Input: part model. Units: mm. Frame: model coordinates. A direction names the side the tool comes from. Round coordinates to 2 decimals unless told otherwise and drop trailing zeros. Order: outer loops, then holes, each group sorted by start corner. A loop starts at its lowest first (then second) coordinate and runs counter-clockwise, first axis right, second up. Notation, with made-up numbers: M 71,-6 L 76,-6 A14 cw 76,1 Z; hole C 73,89 d4. An arc over 180 degrees is marked long. One line per question, with ' | ' between items.
Solid Edge part; units mm, degrees
sketch "Sketch1" plane through (0, 0, 0) normal (0, -1, 0) x (1, 0, 0)
  line L0 (0, 0) -> (9, 0)
  line L1 (9, 0) -> (7.5, 3)
  line L2 (7.5, 3) -> (0, 3)
  dimension "D1" = 9
  dimension "D2" = 7.5
revolve "RevolvedProtrusion1" add sketch "Sketch1" angle 360 about axis through (0, 0, 3) along (0, 0, -1)
sketch "Sketch2" plane through (0, 0, 3) normal (0, 0, 1) x (1, 0, 0)
  line L0 (-0.5, -4) -> (0.5, -4)
  line L1 (0.5, -4) -> (0.5, 4)
  line L2 (0.5, 4) -> (-0.5, 4)
  line L3 (-0.5, 4) -> (-0.5, -4)
  line L4 (1.5, -4) -> (2.5, -4)
  line L5 (2.5, -4) -> (2.5, 4)
  line L6 (2.5, 4) -> (1.5, 4)
  line L7 (1.5, 4) -> (1.5, -4)
  line L8 (-2.5, -4) -> (-1.5, -4)
  line L9 (-1.5, -4) -> (-1.5, 4)
  line L10 (-1.5, 4) -> (-2.5, 4)
  line L11 (-2.5, 4) -> (-2.5, -4)
  dimension "D1" = 0.5
  dimension "D2" = 0.5
extrude "Cutout1" cut sketch "Sketch2" against normal blind 0.5
fillet "main_rounds" radius 0.25 14 edges at (-9, 0, 0) (-7.5, 0, 3) (0.5, 0, 3) (0, -4, 3) (-0.5, 0, 3) (0, 4, 3) (-2.5, 0, 3) (-1.5, 0, 3) (-2, 4, 3) (-2, -4, 3) (2, -4, 3) (1.5, 0, 3) (2.5, 0, 3) (2, 4, 3)
properties material "Polyethylene, low density"
Item 1: First-contact query: pin 1 (0.5 mm diameter, centred on x = -2, y = -2, fed in from +Z); pin 2 (1.5 mm diameter, centred on x = 0, z = 2, fed in from +Y) (3 decimals); pin 3 (10 mm diameter, centred on x = -3, y = 1, fed in from -Z). Flat tips, straight axial feed; report the tip coordinate or a pass-through.
Report:
pin 1: z = 2.5 | pin 2: y = 8.375 | pin 3: z = 0
Item 2: Mould query, pull axis X, two halves, no side actions, for faces 1 (the flat face through (-2, 0, 2.5)), 2 (the conical face through (7.29, -2.3, 2.71)), 3 (the flat face through (0, 0, 0)), 4 (the flat face through (2, 0, 2.5)). Classes: +X half, -X half, draft (parallel to the pull), parting line (faces both ways), or undercut.
Report:
face 1: undercut | face 2: parting line | face 3: draft | face 4: undercut
Item 3: Section query B-B, the plane x = 0. Return loops of the section in (y, z), plus the area to 3 significant figures.
Report:
outline: M -8.82,0.36 A0.25 ccw -8.6,0 L 8.6,0 A0.25 ccw 8.82,0.36 L 7.57,2.86 A0.25 ccw 7.35,3 L 4.25,3 A0.25 ccw 4,2.75 L 4,2.5 L -4,2.5 L -4,2.75 A0.25 ccw -4.25,3 L -7.35,3 A0.25 ccw -7.57,2.86 Z | area: 45.4 mm²
Item 4: Line query: line 1 along X through (y, z) = (-0.5, 2.55); line 2 along Z through (x, y) = (1.75, 1); line 3 along Y through (x, z) = (-1.5, 2.25). Output: solid intervals per line, ascending. Write a range as from..to.
Report:
line 1: -7.71..-2.5, -1.5..-0.5, 0.5..1.5, 2.5..7.71 | line 2: 0..2.5 | line 3: -7.73..7.73
Item 5: Access query for faces 5 (the flat face through (0, 0, 2.5)), 6 (the flat face through (3, 0, 3)). Directions: +Z, -Z, +X, -X, +Y, -Y. A direction counts if a zero-diameter tool reaches every point of the face in a straight line with its end or side. Return the directions, or none.
Report:
face 5: +Z | face 6: +Z, +X, -X, +Y, -Y
Item 6: Section query C-C, the plane z = 1.5. Return loops of the section in (x, y).
Report:
outline: C 0,0 d16.5
Item 7: Section query A-A, the plane y = 0. Return loops of the section in (x, z).
Report:
outline: M -8.82,0.36 A0.25 ccw -8.6,0 L 8.6,0 A0.25 ccw 8.82,0.36 L 7.57,2.86 A0.25 ccw 7.35,3 L 2.75,3 A0.25 ccw 2.5,2.75 L 2.5,2.5 L 1.5,2.5 L 1.5,2.75 A0.25 ccw 1.25,3 L 0.75,3 A0.25 ccw 0.5,2.75 L 0.5,2.5 L -0.5,2.5 L -0.5,2.75 A0.25 ccw -0.75,3 L -1.25,3 A0.25 ccw -1.5,2.75 L -1.5,2.5 L -2.5,2.5 L -2.5,2.75 A0.25 ccw -2.75,3 L -7.35,3 A0.25 ccw -7.57,2.86 Z
